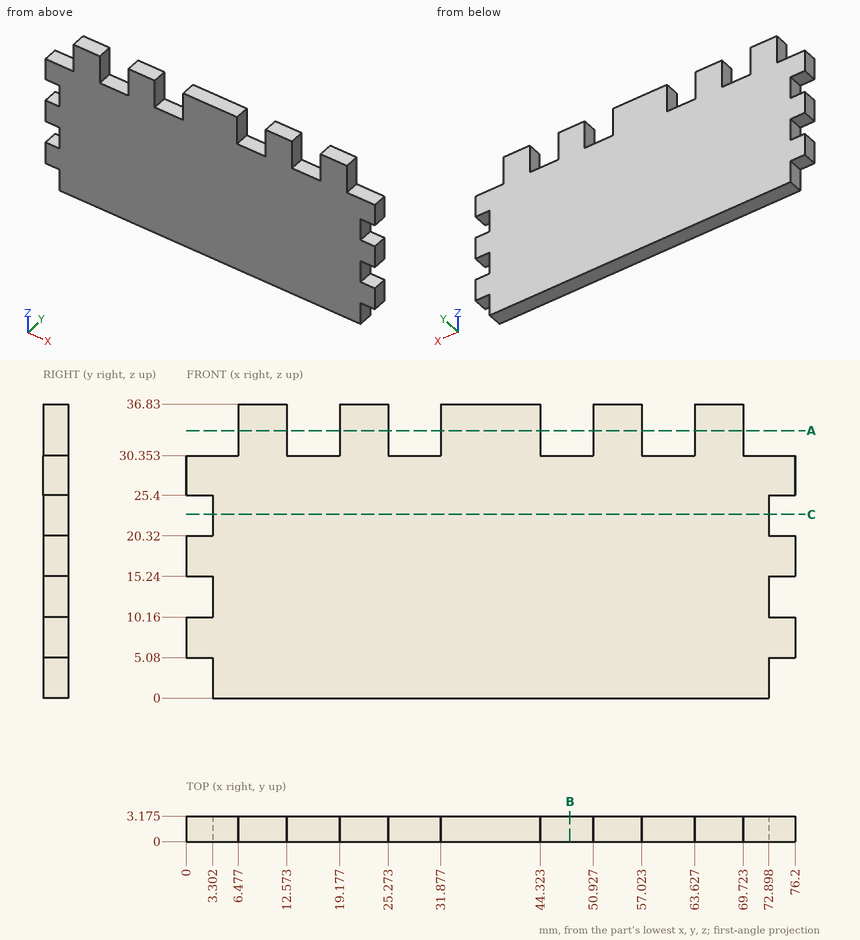
Verification items for this drawing (mm, ordinates from the low corner). Coordinates: 2 decimals unless noted, no trailing zeros. Loops run counter-clockwise (first coordinate to the right, second up) from the corner with the lowest first, then second, coordinate; pieces in that order, holes last. Notation, with made-up numbers: (68.5, -0.75) - (122.5, -0.75) arc R27 ccw to (122.5, 15.25) - close; hole circle Ø10 at (83, -34.75). An arc over 180 degrees is marked (long way). One line per item, written item: value. Start each with the question number.
(1) Material ranges on line 1 (X direction, y = 0.85, z = 35); line 2 (X direction, y = 1.45, z = 13.5); line 3 (Z direction, x = 72, y = 1.6), recorded low to high. Write a range as [from, to].
(2) Cross-section at A-A on z = 33.5. Enter the section's corners in (x, y) (3 decimals).
(3) Depth check by flat-ended pin: P1, Ø12, axis at x = 19.5, z = 9.5, coming from the -Y side; P2, Ø1.6, axis at x = 2.5, y = 1, coming from the +Z side; P3, Ø1, axis at y = 1, z = 33.5, coming from the +X side; P4, Ø1, axis at x = 75.5, y = 1.5, coming from the -Z side. Enter the tip coordinate at first touch or a pass-through.
(4) Cross-section at B-B on x = 48. Enter the section's corners in (y, z) (3 decimals), plus the area to 3 significant figures.
(5) Cross-section at C-C on z = 23. Enter the section's corners in (x, y) (3 decimals).
Results below:
1. line 1: x = [6.48, 12.57], [19.18, 25.27], [31.88, 44.32], [50.93, 57.02], [63.63, 69.72]
1. line 2: x = [3.3, 72.9]
1. line 3: z = [0, 30.35]
2. outline: (6.477, 0) - (12.573, 0) - (12.573, 3.175) - (6.477, 3.175) - close; (19.177, 0) - (25.273, 0) - (25.273, 3.175) - (19.177, 3.175) - close; (31.877, 0) - (44.323, 0) - (44.323, 3.175) - (31.877, 3.175) - close; (50.927, 0) - (57.023, 0) - (57.023, 3.175) - (50.927, 3.175) - close; (63.627, 0) - (69.723, 0) - (69.723, 3.175) - (63.627, 3.175) - close
3. P1: stops at y = 0
3. P2: stops at z = 30.35
3. P3: stops at x = 69.72
3. P4: stops at z = 5.08
4. outline: (0, 0) - (3.175, 0) - (3.175, 30.353) - (0, 30.353) - close
4. area: 96.4 mm2
5. outline: (3.302, 0) - (72.898, 0) - (72.898, 3.175) - (3.302, 3.175) - close
